Could you check a few things on this model? Use its own coordinates, in mm. Face numbers are marked on the shaded views. A direction names the side the tool comes from. Give positions to 0.01 mm unless a question says otherwise; leave off trailing zeros. Order: outer loops, then holes, each group sorted by start corner. A loop starts at its lowest first (then second) coordinate and runs counter-clockwise, first axis right, second up. Notation, with made-up numbers: (39, 72.5) - (75, 72.5) arc R19 ccw to (75, 108.5) - close; hole circle Ø5 at (7, -32.5). An arc over 180 degrees is marked (long way). One line per question, with ' | ' between items. Start each with the question number.
1. If we mould it in two halves opening along X, with no side actions, what happens to the marked faces 4, 5, 6 and 7? For each: released by +X, released by -X, zero draft, split by the parting line, or undercut.
2. Which directions (+Z, -Z, +X, -X, +Y, -Y) give clear straight access to the entire face, cutting with the end or side of a thin tool? Please do the marked faces 1, 2 and 3.
3. Imagine slicing it at B-B (z = 3.25). Please give me the cut outline in (x, y), and give its area (3 significant figures).
4. Imagine slicing it at D-D (z = 14.25). Please give me the cut outline in (x, y).
5. I need wall thicknesses on probe 1 along X at (y, z) = (3.75, 1.25); probe 2 along Y at (x, z) = (-10.6, 11.43); probe 3 along X at (y, z) = (-2, 3). Which ranges of each line are inside material? Lowest first, please. Write a range as from..to.
6. For P1, Ø4.5, axis at y = 0, z = 11.43, coming from the -X side; P2, Ø0.9, axis at y = 0.5, z = 11, coming from the +X side; P3, Ø1, axis at x = -12, z = 7, coming from the -Y side, each with a flat end and sliding along its axis, tell me the tip position at first contact or that it passes through.
7. Imagine slicing it at A-A (y = 0). Please give me the cut outline in (x, z).
8. Imagine slicing it at C-C (x = -22). Please give me the cut outline in (y, z), and give its area (3 significant figures).
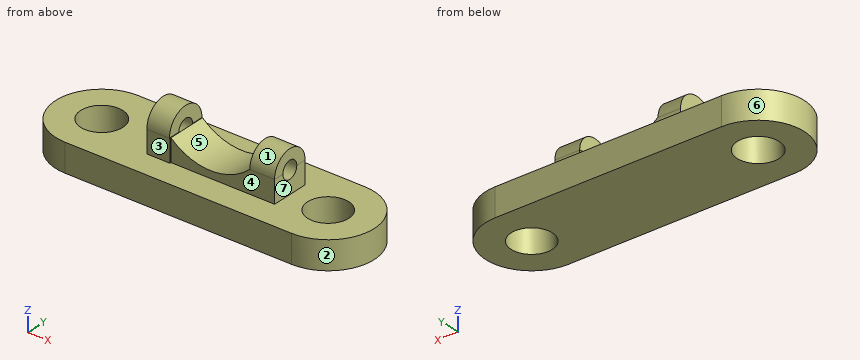
```python
from build123d import *

# Parameters (mm, degrees)
F0_W        = 51.033404
F0_H        = 20.759352
F1_DEPTH    = 25.4
F2_R        = 4.64909
F2_R_2      = 4.755167
F3_DEPTH    = 50.8
F1_FACE_R   = 4.755167
F1_FACE_R_2 = 4.64909
F4_DEPTH    = 19.05
F5_W        = 5.189838
F5_H        = 9.226378
F5_W_2      = 5.766489
F5_H_2      = 8.64973
F6_DEPTH    = 5.08
F8_DEPTH    = 5.08
F10_DEPTH   = 5.588
F11_R       = 1.96352
F12_DEPTH   = 50.8
F13_W       = 17.587781
F13_H       = 8.938054
F14_DEPTH   = 5.08
F16_DEPTH   = 50.8


with BuildPart() as f1:
    # F0 (on Top) → F1 (new body)
    with BuildSketch(Plane.XY):
        with BuildLine():
            ThreePointArc((-25.516702, 10.379676), (-35.896378, 0), (-25.516702, -10.379676))
            Line((-25.516702, -10.379676), (-25.516702, 10.379676))
        make_face()
        Rectangle(F0_W, F0_H)
        with BuildLine():
            Line((25.516702, 10.379676), (25.516702, -10.379676))
            ThreePointArc((25.516702, -10.379676), (35.896378, 0), (25.516702, 10.379676))
        make_face()
    extrude(amount=F1_DEPTH)

    # F2 (on face) → F3 (cut)
    with BuildSketch(Plane.XY.offset(25.4)):
        with Locations((25.516702, 0)):
            Circle(F2_R)
        with Locations((-25.516702, 0)):
            Circle(F2_R_2)
    extrude(amount=-F3_DEPTH, mode=Mode.SUBTRACT)

    # F1_face (on face) → F4 (cut)
    with BuildSketch(Plane.XY.offset(25.4)):
        with BuildLine():
            ThreePointArc((-25.516702, 10.379676), (-35.896378, 0), (-25.516702, -10.379676))
            Line((-25.516702, -10.379676), (25.516702, -10.379676))
            ThreePointArc((25.516702, -10.379676), (35.896378, 0), (25.516702, 10.379676))
            Line((25.516702, 10.379676), (-25.516702, 10.379676))
        make_face()
        with Locations((-25.516702, 0)):
            Circle(F1_FACE_R, mode=Mode.SUBTRACT)
        with Locations((25.516702, 0)):
            Circle(F1_FACE_R_2, mode=Mode.SUBTRACT)
    extrude(amount=-F4_DEPTH, mode=Mode.SUBTRACT)

    # F5 (on face) → F6 (join)
    with BuildSketch(Plane.XY.offset(6.35)):
        with Locations((-9.082216, 0)):
            Rectangle(F5_W, F5_H)
        with Locations((13.983728, 0)):
            Rectangle(F5_W_2, F5_H_2)
    extrude(amount=F6_DEPTH)

    # F7 (on face) → F8 (join)
    with BuildSketch(Plane(origin=(-11.677135, 0, 0), x_dir=(0, -1, 0), z_dir=(-1, 0, 0))):
        with BuildLine():
            Line((-4.613189, 11.43), (4.613189, 11.43))
            ThreePointArc((4.613189, 11.43), (0, 16.043189), (-4.613189, 11.43))
        make_face()
    extrude(amount=-F8_DEPTH)

    # F9 (on face) → F10 (join)
    with BuildSketch(Plane.YZ.offset(16.866973)):
        with BuildLine():
            Line((-4.324865, 11.43), (4.324865, 11.43))
            ThreePointArc((4.324865, 11.43), (0, 15.754865), (-4.324865, 11.43))
        make_face()
    extrude(amount=-F10_DEPTH)

    # F11 (on face) → F12 (cut)
    with BuildSketch(Plane.YZ.offset(16.866973)):
        with Locations((0, 11.43)):
            Circle(F11_R)
    extrude(amount=-F12_DEPTH, mode=Mode.SUBTRACT)

    # F13 (on face) → F14 (join)
    with BuildSketch(Plane.XY.offset(6.35)):
        with Locations((2.306593, 0.144162)):
            Rectangle(F13_W, F13_H)
    extrude(amount=F14_DEPTH)

    # F15 (on face) → F16 (cut)
    with BuildSketch(Plane.XZ.offset(4.324865)):
        with BuildLine():
            Line((11.278973, 11.43), (-6.487297, 11.43))
            ThreePointArc((-6.487297, 11.43), (2.395838, 7.957832), (11.278973, 11.43))
        make_face()
    extrude(amount=-F16_DEPTH, mode=Mode.SUBTRACT)


solid = f1.part
```
Results found:
1) face 4: zero draft | face 5: undercut | face 6: released by -X | face 7: released by +X
2) face 1: +Z, +X | face 2: +Z, -Z, +X | face 3: +Z, +X, -X, -Y
3) outline: (-25.52, -10.38) - (25.52, -10.38) arc R10.38 ccw to (25.52, 10.38) - (-25.52, 10.38) arc R10.38 ccw to start; hole circle Ø9.51 at (-25.52, 0); hole circle Ø9.3 at (25.52, 0) | area: 1,260 mm2
4) outline: (-11.68, -3.65) - (-6.6, -3.65) - (-6.6, 3.65) - (-11.68, 3.65) - close; (11.28, -3.28) - (16.87, -3.28) - (16.87, 3.28) - (11.28, 3.28) - close
5) probe 1: x = -35.2..-28.44, -22.59..22.77, 28.26..35.2 | probe 2: y = -4.61..-1.96, 1.96..4.61 | probe 3: x = -35.7..-29.83, -21.2..21.32, 29.71..35.7
6) P1: stops at x = -11.68 | P2: stops at x = 11.1 | P3: stops at y = -4.61
7) outline: (-35.9, 0) - (-30.27, 0) - (-30.27, 6.35) - (-35.9, 6.35) - close; (-20.76, 0) - (20.87, 0) - (20.87, 6.35) - (16.87, 6.35) - (16.87, 9.47) - (11.1, 9.47) - (11.1, 11.27) arc R13.1 cw to (-6.49, 11.43) - (-6.49, 9.47) - (-11.68, 9.47) - (-11.68, 6.35) - (-20.76, 6.35) - close; (-11.68, 13.39) - (-6.6, 13.39) - (-6.6, 16.04) - (-11.68, 16.04) - close; (11.28, 13.39) - (16.87, 13.39) - (16.87, 15.75) - (11.28, 15.75) - close; (30.17, 0) - (35.9, 0) - (35.9, 6.35) - (30.17, 6.35) - close
8) outline: (-10.38, 0) - (-3.2, 0) - (-3.2, 6.35) - (-10.38, 6.35) - close; (3.2, 0) - (10.38, 0) - (10.38, 6.35) - (3.2, 6.35) - close | area: 91.2 mm2
